Part print with two shaded views. Sizes in mm from the minimum x, y, z corner. A direction names the side the tool comes from. Round coordinates to 2 decimals unless told otherwise and drop trailing zeros. Write each loop counter-clockwise with the first axis right and the second up, starting at its lowest first coordinate (ties: lowest second). Pieces come first, ordered by that corner, then holes. Notation, with made-up numbers: (-1, 60.25) -> (48, 60.25) arc R27 ccw to (48, 85.25) -> close; hole circle Ø7 at (-5.75, 12). An arc over 180 degrees is marked (long way). Answer as CSV lines item,"result".
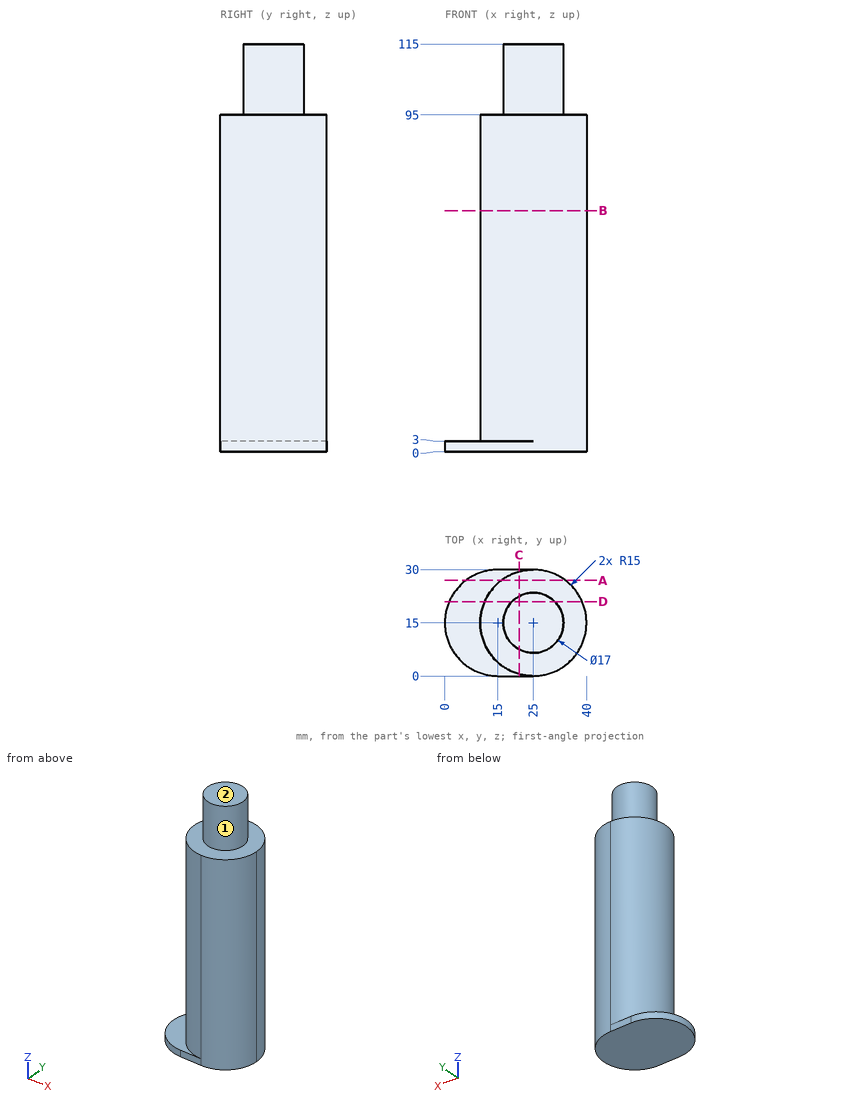
1. Cut at B-B, the plane z = 68. Write the cut outline in (x, y).
Results found:
outline,"(25, 0) arc R15 ccw to (40, 15) arc R15 ccw (long way) to start"
2. Which spindle directions (+Z, -Z, +X, -X, +Y, -Y) get a long thin tool onto all of the face, cutting with end or side? Do the marked faces 1 and 2. Say none if no direction does.
Results found:
face 1,"+Z"
face 2,"+Z, +X, -X, +Y, -Y"
3. Drop flat-ended pins along their axis: pin 1 Ø5 at (y, z) = (3.5, 86) entering from -X; pin 2 Ø2 at (x, z) = (12.5, 24.5) entering from -Y; pin 3 Ø4 at (x, y) = (7.5, 9) entering from +Z. Give the stop position or say it passes through.
Results found:
pin 1,"stops at x = 13"
pin 2,"stops at y = 5.37"
pin 3,"stops at z = 3"
4. Cut at A-A, the plane y = 27. Write the cut outline in (x, z).
Results found:
outline,"(6, 0) -> (34, 0) -> (34, 95) -> (16, 95) -> (16, 3) -> (6, 3) -> close"
5. Cut at C-C, the plane x = 21. Write the cut outline in (y, z).
Results found:
outline,"(0, 0) -> (30, 0) -> (30, 3) -> (29.46, 3) -> (29.46, 95) -> (22.5, 95) -> (22.5, 115) -> (7.5, 115) -> (7.5, 95) -> (0.54, 95) -> (0.54, 3) -> (0, 3) -> close"
6. Cut at D-D, the plane y = 21. Write the cut outline in (x, z).
Results found:
outline,"(1.25, 0) -> (38.75, 0) -> (38.75, 95) -> (31.02, 95) -> (31.02, 115) -> (18.98, 115) -> (18.98, 95) -> (11.25, 95) -> (11.25, 3) -> (1.25, 3) -> close"
7. Probe line 1 along Z through (x, y) = (3, 19); line 2 along Z through (x, y) = (38.5, 20); line 3 along X through (y, z) = (6.5, 37.5). List the from-to ranges inside material, lowest first.
Results found:
line 1,"z = 0 to 3"
line 2,"z = 0 to 95"
line 3,"x = 12.64 to 37.36"
